Verification items for the finished model (mm, model axes). A direction names the side the tool comes from. Give positions to 0.01 mm unless a question says otherwise; leave off trailing zeros. Write each loop counter-clockwise with the first axis right and the second up, starting at its lowest first coordinate (ties: lowest second). Pieces come first, ordered by that corner, then holes. Notation, with made-up numbers: (65, 84.5) - (79, 84.5) arc R30 cw to (79, 114.5) - close; hole circle Ø7 at (-26.75, -11). An arc over 180 degrees is marked (long way). Answer as a JSON object with one key per item and string values. Group by question number.
Item 1: Tool access check on faces 1 (the face through (0, 0, 3)), 2 (the face through (-0.325, 10.536, 12.535)), 3 (the face through (-5, 9, 15)). Record the directions out of +Z, -Z, +X, -X, +Y, -Y that give a thin tool (end or side, any length) a straight path to the whole face; none if there is none.
Item 2: Sectioned sample at C-C, the plane x = 0. Record the boundary of the cut face in (y, z), and give its area (3 significant figures).
Item 3: Go/stop test with flat-tipped pins: pin 1 (5 mm diameter, centred on x = 0, y = -12, fed in from -Z); pin 2 (1.5 mm diameter, centred on x = 0.5, z = 6.5, fed in from +Y); pin 3 (0.9 mm diameter, centred on x = -10, y = 6, fed in from +Z); pin 4 (3 mm diameter, centred on x = -16, y = 2.5, fed in from -Z). Record where each tip stops, or that it passes through.
Item 4: Sectioned sample at A-A, the plane z = 10.5. Record the boundary of the cut face in (x, y), and give its area (3 significant figures).
Item 5: Sectioned sample at B-B, the plane y = 0. Record the boundary of the cut face in (x, z), and give its area (3 significant figures).
Item 6: Draft check along X on faces 4 (the face through (13.887, -10.648, 1.479)), 5 (the face through (-4.336, -19.524, 7.395)), 6 (the face through (0, -18, 0)). Enter one of: +X half, -X half, draft (parallel to the pull), parting line (faces both ways), or undercut.
Item 7: Scan lines: line 1 along Y through (x, z) = (0, 11.7); line 2 along X through (y, z) = (6.5, 14.25); line 3 along Z through (x, y) = (-3, 2.5). Record each from-to range of solid material in increasing order. Write a range as [from, to].
Item 8: Sectioned sample at D-D, the plane x = 7. Record the boundary of the cut face in (y, z) (3 decimals).
```python
from build123d import *

# Parameters (mm, degrees)
SKETCH1_R           = 20
BOSS_EXTRUDE1_DEPTH = 15
SKETCH2_R           = 10
CUT_EXTRUDE1_DEPTH  = 5
SKETCH7_R           = 17.5
CUT_EXTRUDE2_DEPTH  = 3
SKETCH8_R           = 1.5
CUT_EXTRUDE3_DEPTH  = 5


with BuildPart() as part:
    # Sketch1 → Boss-Extrude1 (new body)
    with BuildSketch(Plane.XY):
        Circle(SKETCH1_R)
    extrude(amount=BOSS_EXTRUDE1_DEPTH)

    # Sketch2 → Cut-Extrude1 (cut)
    with BuildSketch(Plane.XY.offset(15)):
        Circle(SKETCH2_R)
    extrude(amount=-CUT_EXTRUDE1_DEPTH, mode=Mode.SUBTRACT)

    # Sketch7 → Cut-Extrude2 (cut)
    with BuildSketch(Plane(origin=(0, 0, 0), x_dir=(-1, 0, 0), z_dir=(0, 0, -1))):
        Circle(SKETCH7_R)
    extrude(amount=-CUT_EXTRUDE2_DEPTH, mode=Mode.SUBTRACT)

    # Sketch8 → Cut-Extrude3 (cut)
    with BuildSketch(Plane.XY.offset(15)):
        with Locations((0, 12)):
            Circle(SKETCH8_R)
        with Locations((10.392304845, 6)):
            Circle(SKETCH8_R)
        with Locations((10.392304845, -6)):
            Circle(SKETCH8_R)
        with Locations((0, -12)):
            Circle(SKETCH8_R)
        with Locations((-10.392304845, -6)):
            Circle(SKETCH8_R)
        with Locations((-10.392304845, 6)):
            Circle(SKETCH8_R)
    extrude(amount=-CUT_EXTRUDE3_DEPTH, mode=Mode.SUBTRACT)


solid = part.part
```
Geometry check:
{
 "1": {"face 1": "-Z", "face 2": "+Z", "face 3": "+Z, +X, -X, +Y, -Y"},
 "2": {"outline": "(-20, 0) - (-17.5, 0) - (-17.5, 3) - (17.5, 3) - (17.5, 0) - (20, 0) - (20, 15) - (13.5, 15) - (13.5, 10) - (10.5, 10) - (10.5, 15) - (10, 15) - (10, 10) - (-10, 10) - (-10, 15) - (-10.5, 15) - (-10.5, 10) - (-13.5, 10) - (-13.5, 15) - (-20, 15) - close", "area": "365 mm^2"},
 "3": {"pin 1": "z = 3", "pin 2": "y = 20", "pin 3": "z = 10", "pin 4": "z = 0"},
 "4": {"outline": "circle Ø40 at (0, 0); hole circle Ø3 at (-10.39, -6); hole circle Ø3 at (-10.39, 6); hole circle Ø20 at (0, 0); hole circle Ø3 at (0, -12); hole circle Ø3 at (0, 12); hole circle Ø3 at (10.39, -6); hole circle Ø3 at (10.39, 6)", "area": "900 mm^2"},
 "5": {"outline": "(-20, 0) - (-17.5, 0) - (-17.5, 3) - (17.5, 3) - (17.5, 0) - (20, 0) - (20, 15) - (10, 15) - (10, 10) - (-10, 10) - (-10, 15) - (-20, 15) - close", "area": "395 mm^2"},
 "6": {"face 4": "undercut", "face 5": "parting line", "face 6": "draft"},
 "7": {"line 1": "[-20, -13.5], [-10.5, -10], [10, 10.5], [13.5, 20]", "line 2": "[-18.91, -11.81], [-8.98, -7.6], [7.6, 8.98], [11.81, 18.91]", "line 3": "[3, 10]"},
 "8": {"outline": "(-18.735, 0) - (-16.039, 0) - (-16.039, 3) - (16.039, 3) - (16.039, 0) - (18.735, 0) - (18.735, 15) - (7.141, 15) - (7.141, 10) - (-7.141, 10) - (-7.141, 15) - (-18.735, 15) - close"}
}
